Model file for the job. Use its own axes, mm. A direction names the side the tool comes from. Coordinates: 2 decimals unless noted, no trailing zeros. Use CSV: the item, a comma, the result in double quotes. Start each with the question number.
from build123d import *

# Parameters (mm, degrees)
BOSS_EXTRUDE1_DEPTH      = 5
CUT_EXTRUDE1_DEPTH       = 23.982085415
BOSS_EXTRUDE3_START      = -5
BOSS_EXTRUDE3_DEPTH      = 5
BOSS_EXTRUDE4_DEPTH      = 10
BOSS_EXTRUDE4_DEPTH_BACK = 15
SKETCH5_W                = 32.55
SKETCH5_H                = 3
SKETCH6_R                = 2.1
CUT_EXTRUDE2_DEPTH       = 10
FILLET1_R                = 5
FILLET2_R                = 1


with BuildPart() as part:
    # Sketch1 → Boss-Extrude1 (new body)
    with BuildSketch(Plane(origin=(0, 0, 0), x_dir=(1, 0, 0), z_dir=(0, 1, 0))):
        with BuildLine():
            Line((0, 12.275), (5, 12.275))
            ThreePointArc((5, 12.275), (6.505980381, 12.009250003), (7.83004518, 11.244101405))
            Line((7.83004518, 11.244101405), (17.20504518, 3.369101405))
            ThreePointArc((17.20504518, 3.369101405), (18.775, 0), (17.20504518, -3.369101405))
            Line((17.20504518, -3.369101405), (7.83004518, -11.244101405))
            ThreePointArc((7.83004518, -11.244101405), (6.505980381, -12.009250003), (5, -12.275))
            Line((5, -12.275), (0, -12.275))
            ThreePointArc((0, -12.275), (-1.505980381, -12.009250003), (-2.83004518, -11.244101405))
            Line((-2.83004518, -11.244101405), (-12.20504518, -3.369101405))
            ThreePointArc((-12.20504518, -3.369101405), (-13.775, 0), (-12.20504518, 3.369101405))
            Line((-12.20504518, 3.369101405), (-2.83004518, 11.244101405))
            ThreePointArc((-2.83004518, 11.244101405), (-1.505980381, 12.009250003), (0, 12.275))
        make_face()
        with BuildLine():
            Line((-9.375, 1.4), (14.375, 1.4))
            ThreePointArc((14.375, 1.4), (15.775, 0), (14.375, -1.4))
            Line((14.375, -1.4), (-9.375, -1.4))
            ThreePointArc((-9.375, -1.4), (-10.775, 0), (-9.375, 1.4))
        make_face(mode=Mode.SUBTRACT)
        with BuildLine():
            Line((0, 9.275), (5, 9.275))
            ThreePointArc((5, 9.275), (6.4, 7.875), (5, 6.475))
            Line((5, 6.475), (0, 6.475))
            ThreePointArc((0, 6.475), (-1.4, 7.875), (0, 9.275))
        make_face(mode=Mode.SUBTRACT)
        with BuildLine():
            Line((0, -6.475), (5, -6.475))
            ThreePointArc((5, -6.475), (6.4, -7.875), (5, -9.275))
            Line((5, -9.275), (0, -9.275))
            ThreePointArc((0, -9.275), (-1.4, -7.875), (0, -6.475))
        make_face(mode=Mode.SUBTRACT)
    extrude(amount=BOSS_EXTRUDE1_DEPTH)

    # Sketch2 → Cut-Extrude1 (cut, through all)
    with BuildSketch(Plane(origin=(0, 5, 0), x_dir=(1, 0, 0), z_dir=(0, 1, 0))):
        with BuildLine():
            Line((0.5, 4), (4.5, 4))
            ThreePointArc((4.5, 4), (8.5, 0), (4.5, -4))
            Line((4.5, -4), (0.5, -4))
            ThreePointArc((0.5, -4), (-3.5, 0), (0.5, 4))
        make_face()
    extrude(amount=-CUT_EXTRUDE1_DEPTH, mode=Mode.SUBTRACT)

    # Sketch4 → Boss-Extrude3 (add)
    with BuildSketch(Plane(origin=(0, 5, 0), x_dir=(1, 0, 0), z_dir=(0, 1, 0)).offset(BOSS_EXTRUDE3_START)):
        with BuildLine():
            Line((-13.775, 0), (-13.775, -20))
            Line((-13.775, -20), (18.775, -20))
            Line((18.775, -20), (18.775, 0))
            ThreePointArc((18.775, 0), (18.363245153, -1.858467273), (17.20504518, -3.369101405))
            Line((17.20504518, -3.369101405), (7.83004518, -11.244101405))
            ThreePointArc((7.83004518, -11.244101405), (6.505980381, -12.009250003), (5, -12.275))
            Line((5, -12.275), (0, -12.275))
            ThreePointArc((0, -12.275), (-1.505980381, -12.009250003), (-2.83004518, -11.244101405))
            Line((-2.83004518, -11.244101405), (-12.20504518, -3.369101405))
            ThreePointArc((-12.20504518, -3.369101405), (-13.363245153, -1.858467273), (-13.775, 0))
        make_face()
    extrude(amount=BOSS_EXTRUDE3_DEPTH)

    # Sketch5 → Boss-Extrude4 (add, two sides: drawn at the far end of the back side and taken through both)
    with BuildSketch(Plane(origin=(0, 5, 0), x_dir=(1, 0, 0), z_dir=(0, 1, 0)).offset(-BOSS_EXTRUDE4_DEPTH_BACK)):
        with Locations((2.5, -18.5)):
            Rectangle(SKETCH5_W, SKETCH5_H)
    extrude(amount=BOSS_EXTRUDE4_DEPTH + BOSS_EXTRUDE4_DEPTH_BACK)

    # Sketch6 → Cut-Extrude2 (cut)
    with BuildSketch(Plane(origin=(0, 0, 17), x_dir=(-1, 0, 0), z_dir=(0, 0, -1))):
        with Locations((-10.5, 11)):
            Circle(SKETCH6_R)
        with Locations((5.5, 11)):
            Circle(SKETCH6_R)
        with Locations(Location((5.5, -6, 0), (0, 0, 180))):
            Circle(SKETCH6_R)
        with Locations(Location((-10.5, -6, 0), (0, 0, 180))):
            Circle(SKETCH6_R)
    extrude(amount=-CUT_EXTRUDE2_DEPTH, mode=Mode.SUBTRACT)

    # Fillet1
    fillet1_edges = [part.edges().sort_by_distance(p)[0] for p in [
        (-13.775, -10, 18.5),
        (18.775, -10, 18.5),
        (-13.775, 15, 18.5),
        (18.775, 15, 18.5),
    ]]
    fillet(fillet1_edges, radius=FILLET1_R)

    # Fillet2
    fillet2_edges = [part.edges().sort_by_distance(p)[0] for p in [
        (18.363245153, 0, -1.858467273),
        (18.363245153, 5, -1.858467273),
        (-13.775, 0, 8.5),
        (-13.775, 5, 8.5),
        (2.5, 0, -12.275),
        (6.505980381, 0, -12.009250003),
        (-13.363245153, 5, -1.858467273),
        (12.51754518, 0, -7.306601405),
        (18.775, 5, 8.5),
        (18.775, 0, 8.5),
        (2.5, 0, 17),
        (2.5, 5, 17),
        (-13.775, 7.5, 17),
        (18.775, 7.5, 17),
        (-13.363245153, 0, -1.858467273),
        (-7.51754518, 0, -7.306601405),
        (-1.505980381, 0, -12.009250003),
        (18.775, -2.5, 17),
        (2.5, -10, 17),
        (-13.775, -2.5, 17),
        (-12.310533906, -8.535533906, 17),
        (17.310533906, -8.535533906, 17),
        (2.5, 15, 17),
        (-12.310533906, 13.535533906, 17),
        (17.310533906, 13.535533906, 17),
        (12.51754518, 5, -7.306601405),
        (6.505980381, 5, -12.009250003),
        (2.5, 5, -12.275),
        (-1.505980381, 5, -12.009250003),
        (-7.51754518, 5, -7.306601405),
    ]]
    fillet(fillet2_edges, radius=FILLET2_R)


solid = part.part
1) Drop flat-ended pins along their axis: P1, Ø4, axis at x = 1, y = 8.5, coming from the -Z side; P2, Ø3, axis at y = 3.5, z = -5, coming from the -X side; P3, Ø12, axis at x = 14, z = 2.5, coming from the +Y side. Give the stop position or say it passes through.
2) Wall check: L1, parallel to Y at x = 10.5, z = 19.2; L2, parallel to X at y = -6, z = 17.85; L3, parallel to Y at x = 10, z = 18. Give the ranges that are in metal, low to high. Write a range as [from, to].
3) Two-plate mould, pull along Z, no slides. Class faces 1 (the face through (12.39, 4.715, -7.021)), 2 (the face through (2, -10, 19)), 3 (the face through (2, 2, 6.475)): pulls with the +Z half, pulls with the -Z half, needs draft (parallel to the pull), parting line crosses it, or undercut.
4) Tool access for faces 4 (the face through (18.474, 4.715, 8.112)), 5 (the face through (-13.474, 4.715, 7.888)), 6 (the face through (2, 0, 5)), 7 (the face through (3, 2, -6.475)): list every direction of +Z, -Z, +X, -X, +Y, -Y with a clear straight run to the whole face (end or side of a thin tool).
5) Band-saw the part on A-A on y = -6. State how many separate pieces and enclosed holes the cut face has, then the cut area to 3 significant figures.
Findings below:
1,P1,"stops at z = 17"
1,P2,"stops at x = -12.05"
1,P3,"stops at y = 5"
2,L1,"y = [-10, -8.1], [-3.9, 8.9], [13.1, 15]"
2,L2,"x = [-13.66, -7.6], [-3.4, 8.4], [12.6, 18.66]"
2,L3,"y = [-10, -8.04], [-3.96, 8.96], [13.04, 15]"
3,face 1,"pulls with the -Z half"
3,face 2,"needs draft"
3,face 3,"undercut"
4,face 4,"-Z, +X, +Y"
4,face 5,"-Z, -X, +Y"
4,face 6,"-Z, +X, -X, -Y"
4,face 7,"+Y, -Y"
5,separate pieces,"3"
5,enclosed holes,"0"
5,area,"71.4 mm2"
